Source: CAD feature listing. Evaluate the final solid. Frame: model axes, mm. Face numbers are marked on the shaded views. A direction names the side the tool comes from. Coordinates: 2 decimals unless noted, no trailing zeros. Write each loop counter-clockwise with the first axis right and the second up, starting at its lowest first coordinate (ties: lowest second). Pieces come first, ordered by that corner, then holes. Notation, with made-up numbers: (15, -38.75) -> (24, -38.75) arc R22 cw to (24, -26.75) -> close; hole circle Ø10 at (20, 30). An arc over 180 degrees is marked (long way). Write item = value, one per line.
from build123d import *

# Parameters (mm, degrees)
F0_W     = 39.6977961063
F0_H     = 55.2159845829
F1_DEPTH = 25.4
F2_SIZE  = 7.62
F3_SIZE  = 5.08
F4_SIZE  = 7.62
F5_DEPTH = 50.8
F6_R     = 7.62


with BuildPart() as f1:
    # F0 (on Front) → F1 (new body)
    with BuildSketch(Plane.XZ):
        with Locations((19.8488980532, 27.6079922915)):
            Rectangle(F0_W, F0_H)
    extrude(amount=F1_DEPTH)

    # F2
    f2_edges = [f1.edges().sort_by_distance(p)[0] for p in [
        (19.848898, -25.4, 55.215985),
        (0, -12.7, 55.215985),
        (39.697796, -12.7, 55.215985),
        (19.848898, 0, 55.215985),
    ]]
    chamfer(f2_edges, length=F2_SIZE)

    # F3
    f3_edges = [f1.edges().sort_by_distance(p)[0] for p in [
        (39.697796, 0, 23.797992),
        (0, -25.4, 23.797992),
        (39.697796, -25.4, 23.797992),
        (0, 0, 23.797992),
    ]]
    chamfer(f3_edges, length=F3_SIZE)

    # F4
    f4_edges = [f1.edges().sort_by_distance(p)[0] for p in [
        (2.54, -2.54, 0),
        (39.697796, -12.7, 0),
        (0, -12.7, 0),
        (2.54, -22.86, 0),
        (19.848898, -25.4, 0),
        (19.848898, 0, 0),
        (37.157796, -2.54, 0),
        (37.157796, -22.86, 0),
    ]]
    chamfer(f4_edges, length=F4_SIZE)

    # F5 (add): a face of the model
    f5_faces = [f1.faces().sort_by_distance(p)[0] for p in [
        (19.8488980532, 0, 27.6079922915),
    ]]
    extrude(f5_faces, amount=F5_DEPTH)

    # F6
    f6_edges = [f1.edges().sort_by_distance(p)[0] for p in [
        (19.848898, 50.8, 7.62),
        (19.848898, 50.8, 47.595985),
        (5.08, 50.8, 27.607992),
        (34.617796, 50.8, 27.607992),
    ]]
    fillet(f6_edges, radius=F6_R)


solid = f1.part
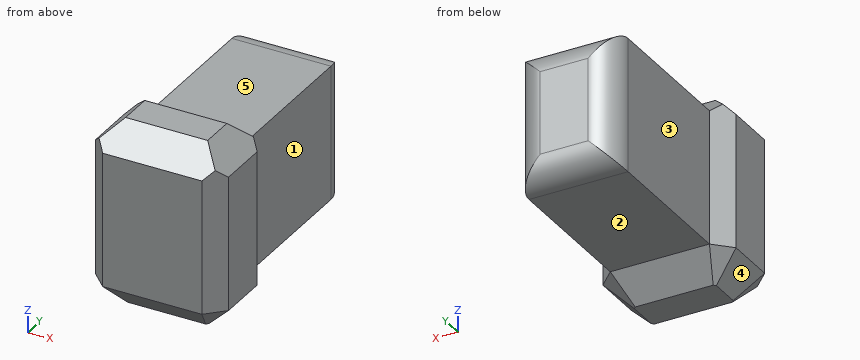
1) Material intervals for probe 1 along Y at (x, z) = (27.5, 30); probe 2 along X at (y, z) = (16, 11); probe 3 along Z at (x, y) = (28, 4), sorted ascending. Write a range as [from, to].
Answer block:
probe_1 = [-25.4, 50.78]
probe_2 = [5.08, 34.62]
probe_3 = [7.62, 47.6]
2) Cut plane A-A, the plane x = 25.5. Output: boundary loops of the cut face in (y, z), and give its area (3 significant figures).
Answer block:
outline = (-25.4, 7.62) -> (-17.78, 0) -> (-7.62, 0) -> (0, 7.62) -> (43.18, 7.62) arc R7.62 ccw to (50.8, 15.24) -> (50.8, 39.98) arc R7.62 ccw to (43.18, 47.6) -> (0, 47.6) -> (-7.62, 55.22) -> (-17.78, 55.22) -> (-25.4, 47.6) -> close
area = 3,290 mm2
3) Cut plane D-D, the plane z = 49. Output: boundary loops of the cut face in (x, y), and give its area (3 significant figures).
Answer block:
outline = (1.4, -21.72) -> (3.68, -24) -> (36.02, -24) -> (38.29, -21.72) -> (38.29, -3.68) -> (36.02, -1.4) -> (3.68, -1.4) -> (1.4, -3.68) -> close
area = 823 mm2
4) First-contact query: pin 1 Ø1 at (x, y) = (10.5, 35) entering from -Z; pin 2 Ø10 at (y, z) = (18, 10.5) entering from -X; pin 3 Ø12 at (x, y) = (11, 40.5) entering from +Z. Flat tips, straight axial feed; report the tip coordinate or a pass-through.
Answer block:
pin_1 = 7.62
pin_2 = 5.08
pin_3 = 47.6
5) Cut plane C-C, the plane y = 7. Output: boundary loops of the cut face in (x, z), and give its area (3 significant figures).
Answer block:
outline = (5.08, 7.62) -> (34.62, 7.62) -> (34.62, 47.6) -> (5.08, 47.6) -> close
area = 1,180 mm2
6) Cut plane B-B, the plane z = 32.5. Output: boundary loops of the cut face in (x, y), and give its area (3 significant figures).
Answer block:
outline = (0, -20.32) -> (5.08, -25.4) -> (34.62, -25.4) -> (39.7, -20.32) -> (39.7, -5.08) -> (34.62, 0) -> (34.62, 43.18) arc R7.62 ccw to (27, 50.8) -> (12.7, 50.8) arc R7.62 ccw to (5.08, 43.18) -> (5.08, 0) -> (0, -5.08) -> close
area = 2,430 mm2
7) Reachability of the marked faces 1, 2, 3, 4 and 5 from +Z, -Z, +X, -X, +Y, -Y: full face, straight path, thin tool, end or side. Return the list, or none.
Answer block:
face_1 = +Z, -Z, +X, +Y
face_2 = -Z, +X, -X, +Y
face_3 = +Z, -Z, -X, +Y
face_4 = -Z, -X, +Y, -Y
face_5 = +Z, +X, -X, +Y
